Could you check a few things on this model? Use its own coordinates, in mm. A direction names the side the tool comes from. Round coordinates to 2 decimals unless told otherwise and drop trailing zeros. Write each loop counter-clockwise with the first axis right and the second up, starting at its lowest first coordinate (ties: lowest second). Pieces come first, ordered by that corner, then holes. Notation, with made-up numbers: (17.25, 32.5) -> (27.25, 32.5) arc R34 ccw to (27.25, 62.5) -> close; hole circle Ø3 at (71, -17.5). An arc over 180 degrees is marked (long way). Answer as CSV lines item,"result". Start each with the question number.
Q1. Imagine slicing it at B-B on y = -2.5. Please give me the cut outline in (x, z), and give its area (4 significant figures).
Q2. Will these pins go through, and if not, where does the flat tip stop? pin 1 Ø1.8 at (y, z) = (0.5, 1.5) entering from -X; pin 2 Ø1 at (x, z) = (-0.5, 5) entering from -Y; pin 3 Ø1.6 at (y, z) = (1.5, 4.5) entering from +X.
Q3. Imagine slicing it at C-C on x = -0.2. Please give me the cut outline in (y, z), and give its area (4 significant figures).
Q4. For faces 1 (the flat face through (-1, 1, 4)), 2 (the flat face through (0, 2.05, 4)), 3 (the flat face through (1, 1, 4)), 4 (the flat face through (0, 0.05, 4)), which set-ups out of +Z, -Z, +X, -X, +Y, -Y let a thin tool reach every point of the face, with its end or its side?
Q5. If I drill on line 1 (Z direction, x = 1.55, y = -0.75); line 2 (Z direction, x = -0.55, y = 1.5); line 3 (Y direction, x = 1.7, z = -1.25), over which ranges is the centre line in solid material (lowest first)? Write a range as [from, to].
Q6. Imagine slicing it at D-D on z = 2. Please give me the cut outline in (x, y), and give its area (4 significant figures).
Q7. Imagine slicing it at A-A on z = -0.75. Please give me the cut outline in (x, y), and give its area (3 significant figures).
Autodesk Inventor part; units mm, degrees
ref_plane "YZ Plane" through (0, 0, 0) normal (1, 0, 0) x (0, 1, 0)
ref_plane "XZ Plane" through (0, 0, 0) normal (0, 1, 0) x (-1, 0, 0)
ref_plane "XY Plane" through (0, 0, 0) normal (0, 0, 1) x (1, 0, 0)
sketch "スケッチ1" plane through (0, 0, 0) normal (0, 0, 1) x (1, 0, 0)
  line L0 (-1.75, -4.25) -> (1.75, -4.25)
  line L1 (1.75, -4.25) -> (1.75, 4.25)
  line L2 (1.75, 4.25) -> (-1.75, 4.25)
  line L3 (-1.75, 4.25) -> (-1.75, -4.25)
  line L4 (-1.75, -4.25) -> (1.75, 4.25) construction
  line L5 (1.75, -4.25) -> (-1.75, 4.25) construction
  point P0 (0, 0)
  dimension "d0" = 3.5
  dimension "d1" = 8.5
extrude "押し出し1" add sketch "スケッチ1" along normal blind 3.5
sketch "スケッチ2" plane through (0, 0, 0) normal (0, 0, -1) x (-1, 0, 0)
  line L0 (1.6, -2.5) -> (-1.6, -2.5) construction
  line L1 (-1.6, -2.5) -> (-1.6, 2.5) construction
  line L2 (-1.6, 2.5) -> (1.6, 2.5) construction
  line L3 (1.6, 2.5) -> (1.6, -2.5) construction
  line L4 (1.6, -2.5) -> (-1.6, 2.5) construction
  line L5 (-1.6, -2.5) -> (1.6, 2.5) construction
  circle A0 centre (-1.6, -2.5) radius 0.25
  point P0 (0, 0)
  dimension "d4" = 3.2
  dimension "d5" = 5
  dimension "d6" = 0.5
extrude "押し出し2" add sketch "スケッチ2" along normal blind 3.1
pattern_linear "矩形状パターン1" count 3 spacing 2.5 along (0, 1, 0) count 2 spacing 3.2 along (-1, 0, 0) of "押し出し2"
sketch "スケッチ3" plane through (0, 0, 3.5) normal (0, 0, 1) x (1, 0, 0)
  line L0 (-1, 0.05) -> (1, 0.05)
  line L1 (1, 0.05) -> (1, 2.05)
  line L2 (1, 2.05) -> (-1, 2.05)
  line L3 (-1, 2.05) -> (-1, 0.05)
  line L4 (-1, 0.05) -> (1, 2.05) construction
  line L5 (1, 0.05) -> (-1, 2.05) construction
  line L6 (1.75, 4.25) -> (-1.75, 4.25)
  point P0 (0, 0)
  point P1 (0, 1.05)
  point P2 (0, 1.05)
  dimension "d15" = 2
  dimension "d16" = 4.2
extrude "押し出し3" add sketch "スケッチ3" along normal blind 2
properties part number "IS-1250"
Checks:
1,outline,"(-1.85, -3.1) -> (-1.35, -3.1) -> (-1.35, 0) -> (1.35, 0) -> (1.35, -3.1) -> (1.85, -3.1) -> (1.85, 0) -> (1.75, 0) -> (1.75, 3.5) -> (-1.75, 3.5) -> (-1.75, 0) -> (-1.85, 0) -> close"
1,area,"15.35 mm^2"
2,pin 1,"x = -1.75"
2,pin 2,"y = 0.05"
2,pin 3,"x = 1"
3,outline,"(-4.25, 0) -> (4.25, 0) -> (4.25, 3.5) -> (2.05, 3.5) -> (2.05, 5.5) -> (0.05, 5.5) -> (0.05, 3.5) -> (-4.25, 3.5) -> close"
3,area,"33.75 mm^2"
4,face 1,"+Z, -X, +Y, -Y"
4,face 2,"+Z, +X, -X, +Y"
4,face 3,"+Z, +X, +Y, -Y"
4,face 4,"+Z, +X, -X, -Y"
5,line 1,"[0, 3.5]"
5,line 2,"[0, 5.5]"
5,line 3,"[-2.73, -2.27], [-0.23, 0.23], [2.27, 2.73]"
6,outline,"(-1.75, -4.25) -> (1.75, -4.25) -> (1.75, 4.25) -> (-1.75, 4.25) -> close"
6,area,"29.75 mm^2"
7,outline,"circle Ø0.5 at (-1.6, -2.5); circle Ø0.5 at (-1.6, 0); circle Ø0.5 at (-1.6, 2.5); circle Ø0.5 at (1.6, -2.5); circle Ø0.5 at (1.6, 0); circle Ø0.5 at (1.6, 2.5)"
7,area,"1.18 mm^2"
